The drawing under review shows one solid part. Ordinate dimensions are in mm from its lowest x, y, z. A direction names the side the tool comes from. Coordinates: 2 decimals unless noted, no trailing zeros. Write each loop counter-clockwise with the first axis right and the second up, starting at its lowest first coordinate (ties: lowest second). Pieces come first, ordered by that corner, then holes. Notation, with made-up numbers: (-19, -1) - (4, -1) arc R31 ccw to (4, 35) - close; hole circle Ø2 at (-22.75, 51.5). An arc over 180 degrees is marked (long way). Put each result on its own line as item: value. Start each with the question number.
Item 1: Consider section C-C on x = 17.5. Give the boundary of the cut face in (y, z), then the cut area to 3 significant figures.
Item 2: To check wall thickness, follow L1, parallel to Y at x = 10, z = 0.85; L2, parallel to Y at x = 10, z = 1.55; L3, parallel to Z at x = 15.75, y = 6.75. State the ranges of each line that lie inside material, in increasing order. Write a range as [from, to].
Item 3: Machinability: for the marked faces 1 and 2, which of the approach directions +Z, -Z, +X, -X, +Y, -Y give a long, thin tool a straight path to every point of the face, cutting with its end or side? Answer none if there is none.
Item 4: For pin 1 (2 mm diameter, centred on x = 7.5, z = 2, fed in from +Y); pin 2 (3.5 mm diameter, centred on x = 3, y = 10, fed in from +Z); pin 3 (1.8 mm diameter, centred on x = 9, y = 9, fed in from +Z), all flat-tipped, find the tip position at first contact; note any pin that passes through.
Item 5: Consider section A-A on x = 10. Give the boundary of the cut face in (y, z).
Item 6: Consider section D-D on y = 3. Give the boundary of the cut face in (x, z).
Item 7: Mouldability with a two-part tool opening along X and no side actions: class the marked faces 3, 4, 5 and 6 as pulls with the +X half, pulls with the -X half, needs draft (parallel to the pull), parting line crosses it, or undercut.
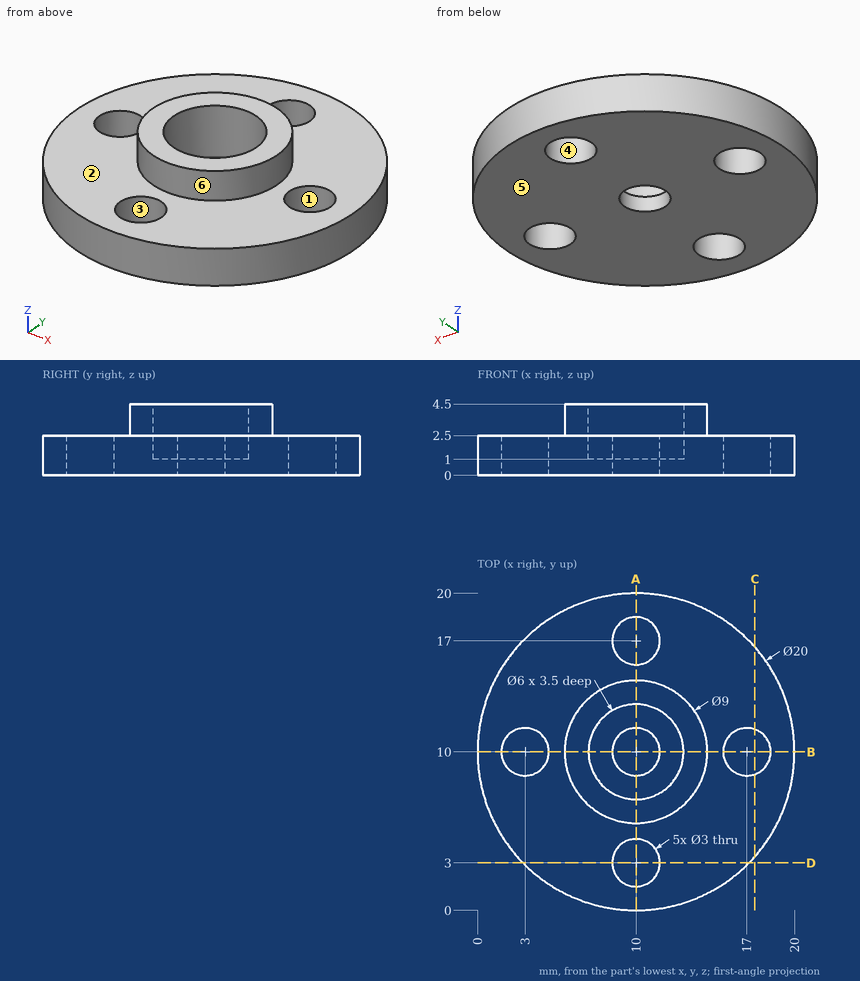
Report:
1. outline: (3.39, 0) - (8.59, 0) - (8.59, 2.5) - (3.39, 2.5) - close; (11.41, 0) - (16.61, 0) - (16.61, 2.5) - (11.41, 2.5) - close
1. area: 26.0 mm²
2. L1: [0, 1.5], [4.5, 8.5], [11.5, 15.5], [18.5, 20]
2. L2: [0, 1.5], [4.5, 7], [13, 15.5], [18.5, 20]
2. L3: [0, 2.5]
3. face 1: +Z, -Z
3. face 2: +Z
4. pin 1: y = 19.89
4. pin 2: z = 2.5
4. pin 3: z = 1
5. outline: (0, 0) - (1.5, 0) - (1.5, 2.5) - (0, 2.5) - close; (4.5, 0) - (8.5, 0) - (8.5, 1) - (7, 1) - (7, 4.5) - (5.5, 4.5) - (5.5, 2.5) - (4.5, 2.5) - close; (11.5, 0) - (15.5, 0) - (15.5, 2.5) - (14.5, 2.5) - (14.5, 4.5) - (13, 4.5) - (13, 1) - (11.5, 1) - close; (18.5, 0) - (20, 0) - (20, 2.5) - (18.5, 2.5) - close
6. outline: (2.86, 0) - (8.5, 0) - (8.5, 2.5) - (2.86, 2.5) - close; (11.5, 0) - (17.14, 0) - (17.14, 2.5) - (11.5, 2.5) - close
7. face 3: undercut
7. face 4: undercut
7. face 5: needs draft
7. face 6: parting line crosses it
